Work out the finished part from the listing and answer in its coordinate system (mm). Face numbers are marked on the shaded views. Coordinates: 2 decimals unless noted, no trailing zeros. Order: outer loops, then holes, each group sorted by start corner. A loop starts at its lowest first (then second) coordinate and runs counter-clockwise, first axis right, second up. Notation, with made-up numbers: (35.5, 3) -> (39.5, 3) arc R29 ccw to (39.5, 40) -> close; hole circle Ø11 at (73.25, -16). An arc over 180 degrees is marked (long way). Use one line per item in the form item = value.
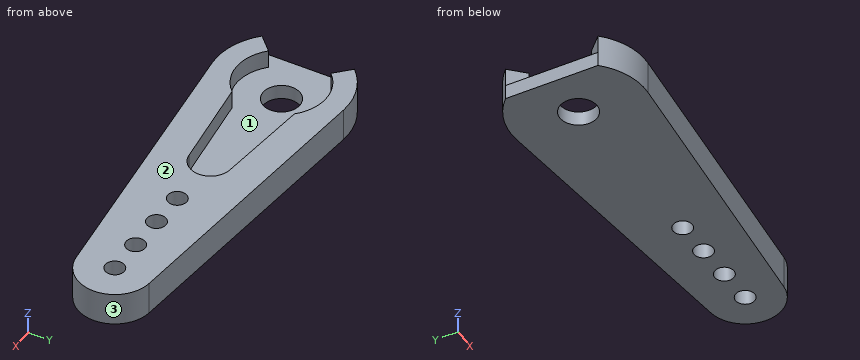
from build123d import *

# Parameters (mm, degrees)
MAIN_DEPTH            = 2.5
ESQUISSE2_R           = 2.5
ORIGINALBRACKET_DEPTH = 2
ESQUISSE3_R           = 1.3
FIXINGHOLE_DEPTH      = 5.5
LPATTERN1_COUNT       = 4
LPATTERN1_PITCH       = 5


with BuildPart() as part:
    # Esquisse1 → Main (new body)
    with BuildSketch(Plane.XY):
        with BuildLine():
            Line((-4.375785644, 4.25), (-6.426543071, 6.300757427))
            ThreePointArc((-6.426543071, 6.300757427), (-3.065415215, 8.461869153), (0.9, 8.954886934))
            Line((0.9, 8.954886934), (40.5, 4.974937186))
            ThreePointArc((40.5, 4.974937186), (45, 0), (40.5, -4.974937186))
            Line((40.5, -4.974937186), (0.9, -8.954886934))
            ThreePointArc((0.9, -8.954886934), (-3.065415215, -8.461869153), (-6.426543071, -6.300757427))
            Line((-6.426543071, -6.300757427), (-4.375785644, -4.25))
            ThreePointArc((-4.375785644, -4.25), (0, -6.1), (4.375785644, -4.25))
            Line((4.375785644, -4.25), (17.31559729, -2.78215714))
            ThreePointArc((17.31559729, -2.78215714), (19.8, 0), (17.31559729, 2.78215714))
            Line((17.31559729, 2.78215714), (4.375785644, 4.25))
            ThreePointArc((4.375785644, 4.25), (0, 6.1), (-4.375785644, 4.25))
        make_face()
    extrude(amount=MAIN_DEPTH)

    # Esquisse2 → OriginalBracket (add)
    with BuildSketch(Plane(origin=(0, 0, 0), x_dir=(-1, 0, 0), z_dir=(0, 0, -1))):
        with BuildLine():
            Line((-0.9, -8.954886934), (-40.5, -4.974937186))
            ThreePointArc((-40.5, -4.974937186), (-45, 0), (-40.5, 4.974937186))
            Line((-40.5, 4.974937186), (-0.9, 8.954886934))
            ThreePointArc((-0.9, 8.954886934), (3.065415215, 8.461869153), (6.426543071, 6.300757427))
            Line((6.426543071, 6.300757427), (6.426543071, -6.300757427))
            ThreePointArc((6.426543071, -6.300757427), (3.065415215, -8.461869153), (-0.9, -8.954886934))
        make_face()
        Circle(ESQUISSE2_R, mode=Mode.SUBTRACT)
    extrude(amount=ORIGINALBRACKET_DEPTH)

    # Esquisse3 → FixingHole (cut, through all)
    with BuildSketch(Plane.XY.offset(2.5)):
        with Locations((40, 0)):
            Circle(ESQUISSE3_R)
    fixinghole = extrude(amount=-FIXINGHOLE_DEPTH, mode=Mode.SUBTRACT)

    # LPattern1: FixingHole ×4
    with Locations(*[(-i * LPATTERN1_PITCH, 0, 0) for i in range(1, LPATTERN1_COUNT)]):
        add(fixinghole, mode=Mode.SUBTRACT)


solid = part.part
(1) Each of these flat-tipped pins is pushed along its axis until it touches: P1, Ø2, axis at y = -4, z = -1.5, coming from the +X side; P2, Ø2, axis at x = 5.5, z = -1, coming from the +Y side; P3, Ø8, axis at x = 0, y = 0, coming from the +Z side. Where does it stop, or does it pass through?
Data:
P1 = 44
P2 = 8.59
P3 = 0
(2) Section A-A on y = 0 is taken. Write down the section's boundary in (x, z).
Data:
outline = (-6.43, -2) -> (-2.5, -2) -> (-2.5, 0) -> (-6.43, 0) -> close; (2.5, -2) -> (23.7, -2) -> (23.7, 2.5) -> (19.8, 2.5) -> (19.8, 0) -> (2.5, 0) -> close; (26.3, -2) -> (28.7, -2) -> (28.7, 2.5) -> (26.3, 2.5) -> close; (31.3, -2) -> (33.7, -2) -> (33.7, 2.5) -> (31.3, 2.5) -> close; (36.3, -2) -> (38.7, -2) -> (38.7, 2.5) -> (36.3, 2.5) -> close; (41.3, -2) -> (45, -2) -> (45, 2.5) -> (41.3, 2.5) -> close
(3) The mould has two halves that part along Y. Classify the marked faces 1, 2 and 3: released by +Y, released by -Y, zero draft, split by the parting line, or undercut.
Data:
face_1 = undercut
face_2 = zero draft
face_3 = split by the parting line
(4) Section C-C on z = -1.5 is taken. Write down the section's boundary in (x, y), plus the area to 3 significant figures.
Data:
outline = (-6.43, -6.3) arc R9 ccw to (0.9, -8.95) -> (40.5, -4.97) arc R5 ccw to (40.5, 4.97) -> (0.9, 8.95) arc R9 ccw to (-6.43, 6.3) -> close; hole circle Ø5 at (0, 0); hole circle Ø2.6 at (25, 0); hole circle Ø2.6 at (30, 0); hole circle Ø2.6 at (35, 0); hole circle Ø2.6 at (40, 0)
area = 666 mm²
(5) Section B-B on x = 0 is taken. Write down the section's boundary in (y, z).
Data:
outline = (-9, -2) -> (-2.5, -2) -> (-2.5, 0) -> (-6.1, 0) -> (-6.1, 2.5) -> (-9, 2.5) -> close; (2.5, -2) -> (9, -2) -> (9, 2.5) -> (6.1, 2.5) -> (6.1, 0) -> (2.5, 0) -> close
(6) Straight lines are drawn through the part: line 1 along X through (y, z) = (0.25, 0.55); line 2 along X through (y, z) = (1, 1.9); line 3 along Y through (x, z) = (0, -1.5). For each, find the intervals that lie inside material, in ascending order.
Data:
line_1 = 19.79 to 23.72, 26.28 to 28.72, 31.28 to 33.72, 36.28 to 38.72, 41.28 to 44.99
line_2 = 19.62 to 24.17, 25.83 to 29.17, 30.83 to 34.17, 35.83 to 39.17, 40.83 to 44.9
line_3 = -9 to -2.5, 2.5 to 9
(7) Section D-D on z = 1.1 is taken. Write down the section's boundary in (x, y), plus the area to 3 significant figures.
Data:
outline = (-6.43, -6.3) arc R9 ccw to (0.9, -8.95) -> (40.5, -4.97) arc R5 ccw to (40.5, 4.97) -> (0.9, 8.95) arc R9 ccw to (-6.43, 6.3) -> (-4.38, 4.25) arc R6.1 cw to (4.38, 4.25) -> (17.32, 2.78) arc R2.8 cw to (17.32, -2.78) -> (4.38, -4.25) arc R6.1 cw to (-4.38, -4.25) -> close; hole circle Ø2.6 at (25, 0); hole circle Ø2.6 at (30, 0); hole circle Ø2.6 at (35, 0); hole circle Ø2.6 at (40, 0)
area = 466 mm²
